For this review, take the finished solid that the model builds, in its own axes (mm). A direction names the side the tool comes from. Coordinates: 2 decimals unless noted, no trailing zeros. Write each loop counter-clockwise with the first axis right and the second up, starting at its lowest first coordinate (ties: lowest second). Pieces come first, ordered by that corner, then holes.
1) We need section A-A on z = -13. Write out the cut boundary in (x, y).
2) Insertion check: P1, Ø2, axis at y = -24, z = -29, coming from the -X side; P2, Ø16.5, axis at x = 125, y = 6, coming from the +Z side; P3, Ø8, axis at x = 127.5, z = 0, coming from the +Y side; P4, Ø8, axis at y = -63.5, z = 86, coming from the +X side. Each pin has a flat end and moves straight along its axis. Give the tip position at first contact, or say it passes through.
3) Mouldability with a two-part tool opening along X and no side actions: class faces 5 (the face through (78.1, -54.44, 17.34)), 6 (the face through (45.636, -7.605, 59.517)), 7 (the face through (25, -15, 78)) as pulls with the +X half, pulls with the -X half, needs draft (parallel to the pull), parting line crosses it, or undercut.
4) We need section B-B on x = 25. Write out the cut boundary in (y, z), then the cut area to 3 significant figures.
5) We need section D-D on z = 12.5. Write out the cut boundary in (x, y).
6) To check wall thickness, follow line 1 along X through (y, z) = (-10, 0); line 2 along X through (y, z) = (11.5, 0); line 3 along Y through (x, z) = (0, 77.85). State the ranges of each line that lie inside material, in increasing order.
7) For faces 1 (the face through (50, -15, -50)), 2 (the face through (-119, 11, 30)), 3 (the face through (119, 11, -30)), 4 (the face through (50, -30, 50)), list the 3-axis set-ups (+Z, -Z, +X, -X, +Y, -Y) from which the entire face can be reached by the end or side of a thin tool; tool diameter is ignored.
8) We need section C-C on y = -42.5. Write out the cut boundary in (x, z), then the cut area to 3 significant figures.
from build123d import *

# Parameters (mm, degrees)
SKETCH2_R               = 2.5
CUT_EXTRUDE3_DEPTH      = 5
CUT_EXTRUDE4_REACH      = 222.341
CUT_EXTRUDE6_DEPTH      = 205.08331632
CUT_EXTRUDE6_DEPTH_BACK = 205.08331632
SKETCH6_R               = 2.5


with BuildPart() as part:
    # Sketch1 → Revolve1 (revolve)
    with BuildSketch(Plane.XY, mode=Mode.PRIVATE) as revolve1_sk:
        Polygon((-80, -95), (-80, -15), (-120, -15), (-120, 10), (-135, 10), (-135, 15), (-115, 15), (-115, 0), (-75, 0), (-75, -15), (-70, -15), (-70, -30), (-75, -30), (-75, -95), align=None)
    revolve(revolve1_sk.sketch.rotate(Axis((0, -100.5, 0), (0, 1, 0)), 270), axis=Axis((0, -100.5, 0), (0, 1, 0)))

    # Sketch2 → Cut-Extrude3 (cut)
    with BuildSketch(Plane.XZ.offset(-10)):
        with Locations(Location((127.5, 0, 0), (0, 0, 270))):
            Circle(SKETCH2_R)
        with Locations(Location((-127.5, 0, 0), (0, 0, 270))):
            Circle(SKETCH2_R)
    extrude(amount=-CUT_EXTRUDE3_DEPTH, mode=Mode.SUBTRACT)

    # Cut-Extrude4: up to this face of the body (flat: up to its plane)
    cut_extrude4_end = Plane(part.part.faces().sort_by_distance((0, 0, 111.747308807))[0])
    # Sketch3 → Cut-Extrude4 (cut, up to the picked face)
    with BuildSketch(Plane(origin=(0, 15, 0), x_dir=(1, 0, 0), z_dir=(0, 1, 0)), mode=Mode.PRIVATE) as cut_extrude4_sk1:
        with BuildLine():
            Line((-111.018016556, -30), (-131.624465811, -30))
            ThreePointArc((-131.624465811, -30), (0, -135), (131.624465811, -30))
            Line((131.624465811, -30), (111.018016556, -30))
            ThreePointArc((111.018016556, -30), (0, -115), (-111.018016556, -30))
        make_face()
    cut_extrude4_tool1 = split(extrude(cut_extrude4_sk1.sketch, amount=-CUT_EXTRUDE4_REACH, mode=Mode.PRIVATE), bisect_by=cut_extrude4_end, keep=Keep.BOTH, mode=Mode.PRIVATE)
    # Sketch3 → Cut-Extrude4 (cut, up to the picked face)
    with BuildSketch(Plane(origin=(0, 15, 0), x_dir=(1, 0, 0), z_dir=(0, 1, 0)), mode=Mode.PRIVATE) as cut_extrude4_sk2:
        with BuildLine():
            Line((131.624465811, 30), (111.018016556, 30))
            ThreePointArc((111.018016556, 30), (0, 115), (-111.018016556, 30))
            Line((-111.018016556, 30), (-131.624465811, 30))
            ThreePointArc((-131.624465811, 30), (0, 135), (131.624465811, 30))
        make_face()
    cut_extrude4_tool2 = split(extrude(cut_extrude4_sk2.sketch, amount=-CUT_EXTRUDE4_REACH, mode=Mode.PRIVATE), bisect_by=cut_extrude4_end, keep=Keep.BOTH, mode=Mode.PRIVATE)
    add(cut_extrude4_tool1.solids().sort_by(Axis((-121.321241, 15, 32.834167), (0, -1, 0)))[0], mode=Mode.SUBTRACT)
    add(cut_extrude4_tool2.solids().sort_by(Axis((-121.321241, 15, -32.834167), (0, -1, 0)))[0], mode=Mode.SUBTRACT)

    # Sketch6 → Cut-Extrude6 (cut, two sides: drawn at the far end of the back side and taken through both)
    with BuildSketch(Plane.XY.offset(-CUT_EXTRUDE6_DEPTH_BACK)):
        with Locations((0, -60)):
            Circle(SKETCH6_R)
    extrude(amount=CUT_EXTRUDE6_DEPTH + CUT_EXTRUDE6_DEPTH_BACK, mode=Mode.SUBTRACT)


solid = part.part
Result:
1. outline: (-134.37, 10) - (-119.29, 10) - (-119.29, -15) - (-78.94, -15) - (-78.94, -95) - (-73.86, -95) - (-73.86, -30) - (-68.78, -30) - (-68.78, -15) - (-73.86, -15) - (-73.86, 0) - (-114.26, 0) - (-114.26, 15) - (-134.37, 15) - close; (68.78, -30) - (73.86, -30) - (73.86, -95) - (78.94, -95) - (78.94, -15) - (119.29, -15) - (119.29, 10) - (134.37, 10) - (134.37, 15) - (114.26, 15) - (114.26, 0) - (73.86, 0) - (73.86, -15) - (68.78, -15) - close
2. P1: stops at x = -74.94
2. P2: stops at z = 30
2. P3: stops at y = 15
2. P4: passes through
3. face 5: parting line crosses it
3. face 6: undercut
3. face 7: needs draft
4. outline: (-95, -75.99) - (-15, -75.99) - (-15, -117.37) - (0, -117.37) - (0, -70.71) - (-15, -70.71) - (-15, -65.38) - (-30, -65.38) - (-30, -70.71) - (-95, -70.71) - close; (-95, 70.71) - (-30, 70.71) - (-30, 65.38) - (-15, 65.38) - (-15, 70.71) - (0, 70.71) - (0, 117.37) - (-15, 117.37) - (-15, 75.99) - (-95, 75.99) - close
4. area: 2,400 mm2
5. outline: (-134.42, 10) - (-119.35, 10) - (-119.35, -15) - (-79.02, -15) - (-79.02, -95) - (-73.95, -95) - (-73.95, -30) - (-68.87, -30) - (-68.87, -15) - (-73.95, -15) - (-73.95, 0) - (-114.32, 0) - (-114.32, 15) - (-134.42, 15) - close; (68.87, -30) - (73.95, -30) - (73.95, -95) - (79.02, -95) - (79.02, -15) - (119.35, -15) - (119.35, 10) - (134.42, 10) - (134.42, 15) - (114.32, 15) - (114.32, 0) - (73.95, 0) - (73.95, -15) - (68.87, -15) - close
6. line 1: x = -120 to -75, 75 to 120
6. line 2: x = -135 to -130, -125 to -115, 115 to 125, 130 to 135
6. line 3: y = -95 to -62.5, -57.5 to 0
7. face 1: +Y
7. face 2: +Z, +X, -X, +Y
7. face 3: -Z, +X, -X, +Y
7. face 4: -Y
8. outline: circle Ø160 at (0, 0); hole circle Ø150 at (0, 0)
8. area: 2,430 mm2
